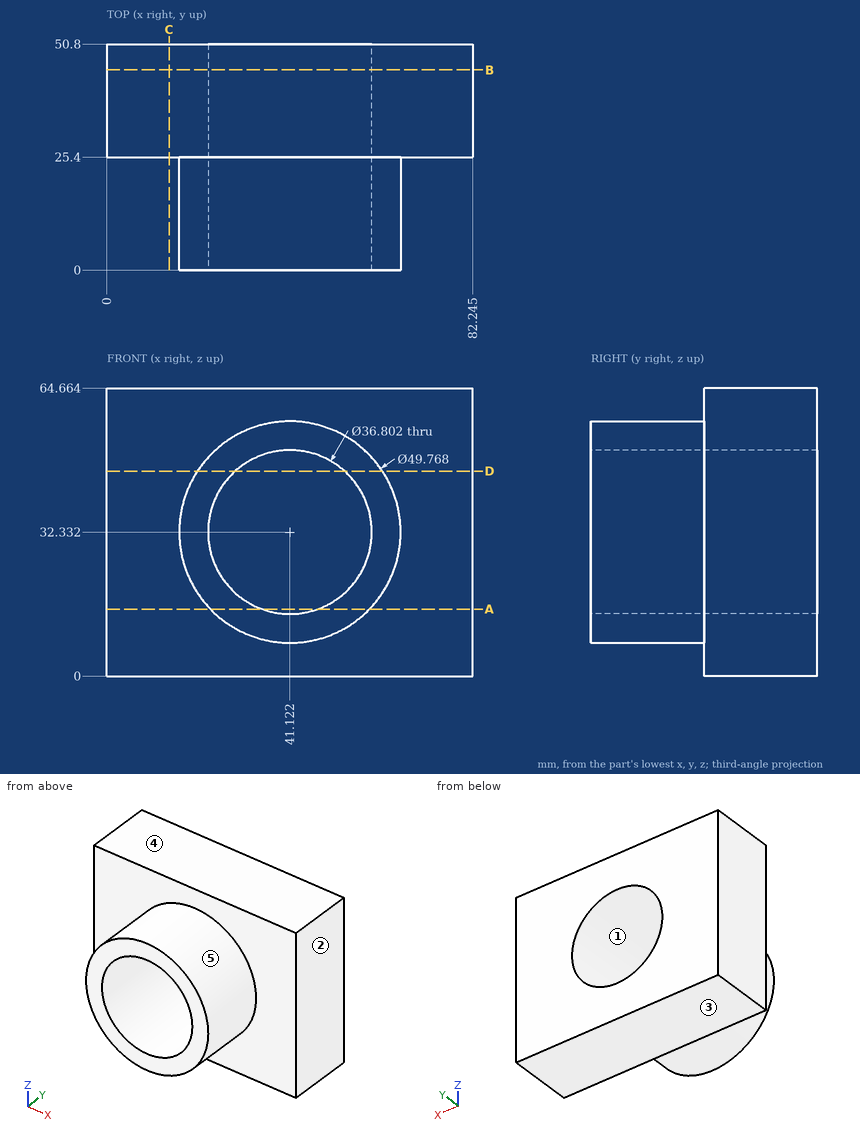
Here's the drawing with two shaded views (mm, measured from the low corner). I have some questions. A direction names the side the tool comes from. Coordinates: 2 decimals unless noted, no trailing zeros. Write each loop counter-clockwise with the first axis right and the second up, starting at its lowest first coordinate (ties: lowest second). Pieces come first, ordered by that corner, then holes. Notation, with made-up numbers: M -23.75,-2 L 19.25,-2 A16 cw 19.25,14 Z; hole C -14.75,10.5 d11. An arc over 180 degrees is marked long. Answer as CSV lines item,"result". Start each with the question number.
1) For P1, Ø10, axis at x = 33, z = 20, coming from the +Y side; P2, Ø5, axis at y = 14.5, z = 7, coming from the -X side (1 decimal); P3, Ø8, axis at x = 66.5, y = 6, coming from the -Z side (1 decimal), each with a flat end and sliding along its axis, tell me the tip position at first contact or that it passes through.
2) I want a section at B-B, the plane y = 45. Please give me the cut outline in (x, z) (1 decimal).
3) Please list where these lines run through material, in increasing order: line 1 (Y direction, x = 5.5, z = 42.5); line 2 (Z direction, x = 27, y = 13) (1 decimal); line 3 (Z direction, x = 37.5, y = 4). Write a range as from..to.
4) I want a section at C-C, the plane x = 14. Please give me the cut outline in (y, z).
5) I want a section at D-D, the plane z = 46. Please give me the cut outline in (x, y) (1 decimal), and give its area (3 significant figures).
6) We'd pull the mould along X, two halves only. Please class the marked faces 1, 2 and 3: +X half, -X half, draft (parallel to the pull), parting line (faces both ways), or undercut.
7) I want a section at A-A, the plane z = 15. Please give me the cut outline in (x, y) (1 decimal).
8) For the marked faces 4 and 5, which set-ups out of +Z, -Z, +X, -X, +Y, -Y let a thin tool reach every point of the face, with its end or its side?
Data:
1,P1,"stops at y = 50.8"
1,P2,"stops at x = 31.2"
1,P3,"stops at z = 19.6"
2,outline,"M 0,0 L 82.2,0 L 82.2,64.7 L 0,64.7 Z; hole C 41.1,32.3 d36.8"
3,line 1,"y = 25.4..50.8"
3,line 2,"z = 11.8..20.5, 44.1..52.8"
3,line 3,"z = 7.71..14.29, 50.37..56.95"
4,outline,"M 25.4,0 L 50.8,0 L 50.8,64.66 L 25.4,64.66 Z"
5,outline,"M 0,25.4 L 20.3,25.4 L 20.3,0 L 28.8,0 L 28.8,50.8 L 0,50.8 Z; M 53.4,0 L 61.9,0 L 61.9,25.4 L 82.2,25.4 L 82.2,50.8 L 53.4,50.8 Z"
5,area,"1,890 mm^2"
6,face 1,"undercut"
6,face 2,"+X half"
6,face 3,"draft"
7,outline,"M 0,25.4 L 23.3,25.4 L 23.3,0 L 34.9,0 L 34.9,50.8 L 0,50.8 Z; M 47.3,0 L 59,0 L 59,25.4 L 82.2,25.4 L 82.2,50.8 L 47.3,50.8 Z"
8,face 4,"+Z, +X, -X, +Y, -Y"
8,face 5,"-Y"
